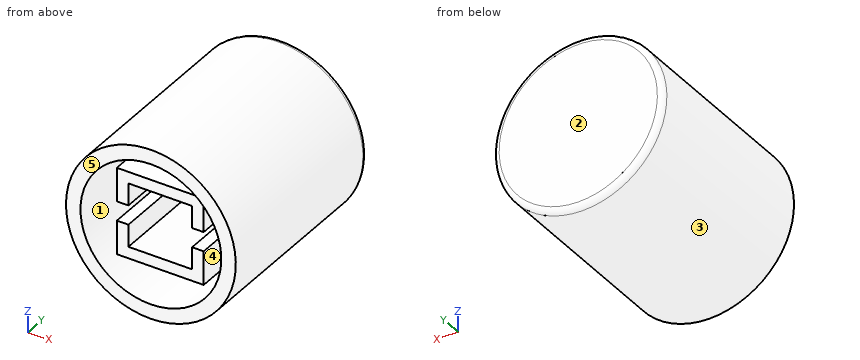
from build123d import *

# Parameters (mm, degrees)
SKETCH1_R           = 4.4
BOSS_EXTRUDE1_DEPTH = 10.5
SHELL1_T            = -0.75
SKETCH3_W           = 4.5
SKETCH3_H           = 4.5
SKETCH3_W_2         = 3.3
SKETCH3_H_2         = 3.3
BOSS_EXTRUDE2_DEPTH = 9
SKETCH5_W           = 4.5
SKETCH5_H           = 1
CUT_EXTRUDE1_DEPTH  = 6.4
FILLET1_R           = 0.3


with BuildPart() as part:
    # Sketch1 → Boss-Extrude1 (new body)
    with BuildSketch(Plane(origin=(0, 0, 0), x_dir=(1, 0, 0), z_dir=(0, 1, 0))):
        with Locations(Location((0, 0, 0), (0, 0, 90))):
            Circle(SKETCH1_R)
    extrude(amount=BOSS_EXTRUDE1_DEPTH)

    # Shell1
    shell1_openings = [part.faces().sort_by_distance(p)[0] for p in [
        (0, 0, 0),
    ]]
    offset(amount=SHELL1_T, openings=shell1_openings, kind=Kind.INTERSECTION)

    # Sketch3 → Boss-Extrude2 (add)
    with BuildSketch(Plane.XZ.offset(-9.75)):
        Rectangle(SKETCH3_W, SKETCH3_H)
        Rectangle(SKETCH3_W_2, SKETCH3_H_2, mode=Mode.SUBTRACT)
    extrude(amount=BOSS_EXTRUDE2_DEPTH)

    # Sketch5 → Cut-Extrude1 (cut)
    with BuildSketch(Plane(origin=(0, 0.75, 0), x_dir=(-1, 0, 0), z_dir=(0, -1, 0))):
        Rectangle(SKETCH5_W, SKETCH5_H)
    extrude(amount=-CUT_EXTRUDE1_DEPTH, mode=Mode.SUBTRACT)

    # Fillet1
    fillet1_edges = [part.edges().sort_by_distance(p)[0] for p in [
        (0, 10.5, 4.4),
    ]]
    fillet(fillet1_edges, radius=FILLET1_R)


solid = part.part
Input: part model. Units: mm. Frame: model coordinates. Face numbers are marked on the shaded views. A direction names the side the tool comes from. Round coordinates to 2 decimals unless told otherwise and drop trailing zeros. Write each loop counter-clockwise with the first axis right and the second up, starting at its lowest first coordinate (ties: lowest second). Pieces come first, ordered by that corner, then holes.
1) Cut plane B-B (x = 0). Return the cut outline in (y, z).
2) Draft query along Z for the marked faces 1, 2 and 3. Return one class per face: pulls with the +Z half, pulls with the -Z half, needs draft (parallel to the pull), parting line crosses it, or undercut.
3) Cut plane C-C (z = 0). Return the cut outline in (x, y).
4) Reachability of the marked faces 4 and 5 from +Z, -Z, +X, -X, +Y, -Y: full face, straight path, thin tool, end or side. Return the list, or none.
5) Ray query, L1, parallel to X at y = 7.75, z = 0; L2, parallel to X at y = 4, z = 0; L3, parallel to Z at x = 1, y = 5. Return the intervals inside material, ascending.
6) Cut plane A-A (y = 7). Return the cut outline in (x, z).
7) Contact query for flat-ended pins moving along their axis: P1, Ø2, axis at x = -0.5, z = -1.5, coming from the -Y side; P2, Ø0.5, axis at x = 2, y = 4, coming from the +Z side; P3, Ø1, axis at y = 7.5, z = 2, coming from the -X side. Output: stop coordinate, or through.
Geometry says:
1. outline: (0, -4.4) - (10.2, -4.4) arc R0.3 ccw to (10.5, -4.1) - (10.5, 4.1) arc R0.3 ccw to (10.2, 4.4) - (0, 4.4) - (0, 3.65) - (9.75, 3.65) - (9.75, 2.25) - (0.75, 2.25) - (0.75, 1.65) - (9.75, 1.65) - (9.75, -1.65) - (0.75, -1.65) - (0.75, -2.25) - (9.75, -2.25) - (9.75, -3.65) - (0, -3.65) - close
2. face 1: undercut
2. face 2: needs draft
2. face 3: parting line crosses it
3. outline: (-4.4, 0) - (-3.65, 0) - (-3.65, 9.75) - (-2.25, 9.75) - (-2.25, 7.15) - (-1.65, 7.15) - (-1.65, 9.75) - (1.65, 9.75) - (1.65, 7.15) - (2.25, 7.15) - (2.25, 9.75) - (3.65, 9.75) - (3.65, 0) - (4.4, 0) - (4.4, 10.2) arc R0.3 ccw to (4.1, 10.5) - (-4.1, 10.5) arc R0.3 ccw to (-4.4, 10.2) - close
4. face 4: -Y
4. face 5: +Z, -Z, +X, -X, -Y
5. L1: x = -4.4 to -3.65, -2.25 to -1.65, 1.65 to 2.25, 3.65 to 4.4
5. L2: x = -4.4 to -3.65, 3.65 to 4.4
5. L3: z = -4.28 to -3.51, -2.25 to -1.65, 1.65 to 2.25, 3.51 to 4.28
6. outline: circle Ø8.8 at (0, 0); (-2.25, -2.25) - (2.25, -2.25) - (2.25, -0.5) - (1.65, -0.5) - (1.65, -1.65) - (-1.65, -1.65) - (-1.65, -0.5) - (-2.25, -0.5) - close; (-2.25, 0.5) - (-1.65, 0.5) - (-1.65, 1.65) - (1.65, 1.65) - (1.65, 0.5) - (2.25, 0.5) - (2.25, 2.25) - (-2.25, 2.25) - close; hole circle Ø7.3 at (0, 0)
7. P1: stops at y = 0.75
7. P2: stops at z = 4.04
7. P3: stops at x = -4.14
